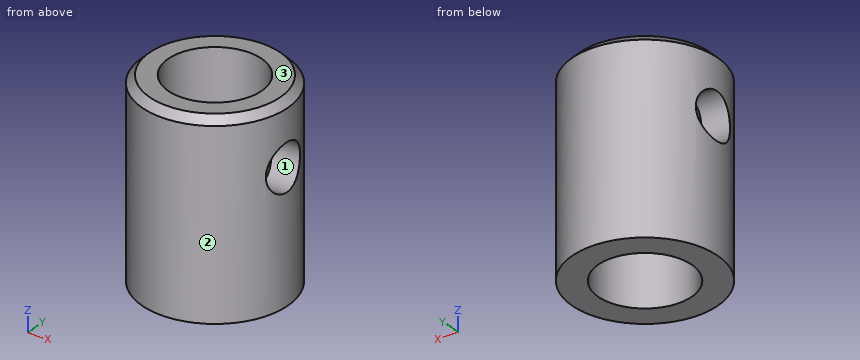
Autodesk Inventor part; units mm, degrees
ref_plane "YZ Plane" through (0, 0, 0) normal (1, 0, 0) x (0, 1, 0)
ref_plane "XZ Plane" through (0, 0, 0) normal (0, 1, 0) x (-1, 0, 0)
ref_plane "XY Plane" through (0, 0, 0) normal (0, 0, 1) x (1, 0, 0)
sketch "Sketch1" plane through (0, 0, 0) normal (0, 0, 1) x (1, 0, 0)
  line L0 (-20.7493, 0) -> (20.7493, 0)
  line L1 (0, -20.7493) -> (0, 20.7493)
  circle A0 centre (0, 0) radius 14.8209
  circle A1 centre (0, 0) radius 9.525
  dimension "d2" = 29.6418
  dimension "d3" = 19.05
extrude "Extrusion1" add sketch "Sketch1" against normal blind 39.116 contours A1 L1 A0 L0 | L0 A0 L1 A1 | A1 L0 A0 L1 | L1 A0 L0 A1
chamfer "Chamfer1" distance 1.524 angle 45 1 edges at (-14.8209, 0, 0) measured on face at (14.7728, -1.1926, -26.0773)
sketch "Sketch2" plane through (0, 0, 0) normal (1, 0, 0) x (0, 1, 0)
  line L0 (-14.8209, -39.116) -> (14.8209, -39.116)
  line L1 (14.8209, -1.524) -> (14.8209, -39.116)
  circle A0 centre (0, -12.7) radius 4.7625
  point P0 (0, 0)
  dimension "d9" = 26.416
  dimension "d10" = 9.525
extrude "Extrusion2" cut sketch "Sketch2" along normal through all both and the other way through all
properties part number "Ch7(5) Part 5 Sleeve"
Input: part model. Units: mm. Frame: model coordinates. Face numbers are marked on the shaded views. Coordinates: 2 decimals unless noted, no trailing zeros. Loops run counter-clockwise (first coordinate to the right, second up) from the corner with the lowest first, then second, coordinate; pieces in that order, holes last.
(1) Section B-B on x = 0. Return the cut outline in (y, z) (3 decimals).
(2) Section D-D on z = -5.5. Return the cut outline in (x, y) (3 decimals), then the cut area to 3 significant figures.
(3) Material intervals for probe 1 along X at (y, z) = (0, -29) (3 decimals); probe 2 along Z at (x, y) = (10, 0); probe 3 along X at (y, z) = (6.25, -18), sorted ascending.
(4) Pull-direction query (Y, two-part tool) for the marked faces 1, 2 and 3; classes: released by +Y, released by -Y, zero draft, split by the parting line, or undercut.
(5) Section A-A on y = 0. Return the cut outline in (x, z) (1 decimal).
(6) First-contact query: pin 1 Ø12 at (x, z) = (-10, -32) entering from -Y; pin 2 Ø3 at (y, z) = (-9, -21.5) entering from +X; pin 3 Ø5 at (y, z) = (1, -16.5) entering from -X; pin 4 Ø2 at (x, z) = (9, -27) entering from +Y. Flat tips, straight axial feed; report the tip coordinate or a pass-through.
Data:
1. outline: (-14.821, -39.116) - (-9.525, -39.116) - (-9.525, 0) - (-13.297, 0) - (-14.821, -1.524) - close; (9.525, -39.116) - (14.821, -39.116) - (14.821, -1.524) - (13.297, 0) - (9.525, 0) - close
2. outline: circle Ø29.642 at (0, 0); hole circle Ø19.05 at (0, 0)
2. area: 405 mm2
3. probe 1: x = -14.821 to -9.525, 9.525 to 14.821
3. probe 2: z = -39.12 to -17.46, -7.94 to 0
3. probe 3: x = -13.44 to -7.19, 7.19 to 13.44
4. face 1: undercut
4. face 2: split by the parting line
4. face 3: zero draft
5. outline: (-14.8, -39.1) - (-9.5, -39.1) - (-9.5, -17.5) - (-14.8, -17.5) - close; (-14.8, -7.9) - (-9.5, -7.9) - (-9.5, 0) - (-13.3, 0) - (-14.8, -1.5) - close; (9.5, -39.1) - (14.8, -39.1) - (14.8, -17.5) - (9.5, -17.5) - close; (9.5, -7.9) - (14.8, -7.9) - (14.8, -1.5) - (13.3, 0) - (9.5, 0) - close
6. pin 1: stops at y = -14.27
6. pin 2: stops at x = 12.78
6. pin 3: stops at x = -14.82
6. pin 4: stops at y = 12.48
